Geometry check sheet. Reference: the model listing, model coordinates, mm. Coordinates: 2 decimals unless noted, no trailing zeros. Order: outer loops, then holes, each group sorted by start corner. A loop starts at its lowest first (then second) coordinate and runs counter-clockwise, first axis right, second up. Notation, with made-up numbers: (37.25, 3) - (60.25, 3) arc R23 ccw to (60.25, 22) - close; hole circle Ø6 at (-3, -16). An arc over 180 degrees is marked (long way). Use CSV: the item, a comma, the result in double quotes. Start each with the question number.
1) Sectioned sample at A-A, the plane z = 0. Record the cut outline in (x, y).
2) Sectioned sample at C-C, the plane x = 9.5. Record the cut outline in (y, z).
3) Sectioned sample at B-B, the plane x = -6.5. Record the cut outline in (y, z).
4) Depth check by flat-ended pin: P1, Ø3, axis at y = -1, z = 7, coming from the +X side; P2, Ø1, axis at y = 0.5, z = 4, coming from the -X side; P3, Ø6, axis at x = 16, z = 3, coming from the +Y side. Enter the tip coordinate at first touch or a pass-through.
5) Sectioned sample at D-D, the plane z = -7.25. Record the cut outline in (x, y).
6) Thickness scan on probe 1 along Y at (x, z) = (-42.75, -4.4); probe 2 along X at (y, z) = (-2.25, 3.5); probe 3 along X at (y, z) = (0.75, 4.25). Record the ranges inside material, lowest first. Write a range as [from, to].
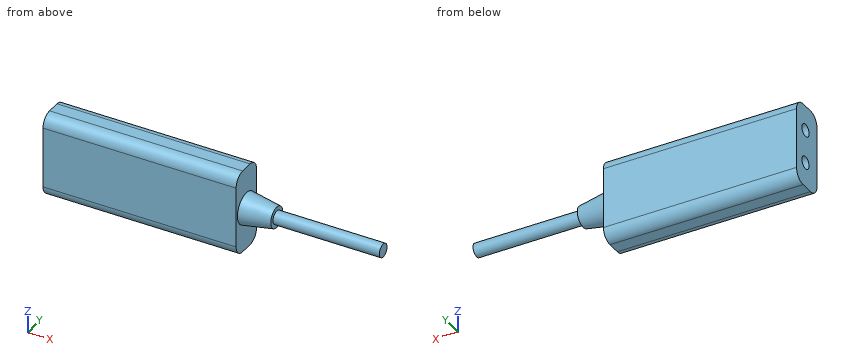
from build123d import *

# Parameters (mm, degrees)
SKETCH_1_W          = 22
SKETCH_1_H          = 9.4
EXTRUDE_1_DEPTH     = 50.8
FILLET_1_R          = 3
SKETCH_4_R          = 1.65
CUT_EXTRUDE_1_DEPTH = 10


with BuildPart() as part:
    # Эскиз1 → Бобышка-Вытянуть1 (new body)
    with BuildSketch(Plane(origin=(0, 0, 0), x_dir=(0, 0, -1), z_dir=(1, 0, 0))):
        Rectangle(SKETCH_1_W, SKETCH_1_H)
    extrude(amount=-EXTRUDE_1_DEPTH)

    # Эскиз3 → Повернуть1 (revolve)
    with BuildSketch(Plane(origin=(0, 0, 0), x_dir=(1, 0, 0), z_dir=(0, 1, 0))):
        Polygon((8, 2.75), (0, 4.1), (0, 0), (36, 0), (36, 1.75), (8, 1.75), align=None)
    revolve(axis=Axis((0, 0, 0), (1, 0, 0)))

    # Скругление1
    fillet_1_edges = [part.edges().sort_by_distance(p)[0] for p in [
        (-25.4, -4.7, 11),
        (-25.4, 4.7, 11),
        (-25.4, 4.7, -11),
        (-25.4, -4.7, -11),
    ]]
    fillet(fillet_1_edges, radius=FILLET_1_R)

    # Эскиз4 → Вырез-Вытянуть1 (cut)
    with BuildSketch(Plane.ZY.offset(50.8)):
        with Locations((-4.4, 0.6)):
            Circle(SKETCH_4_R)
        with Locations((4.4, 0.6)):
            Circle(SKETCH_4_R)
    extrude(amount=-CUT_EXTRUDE_1_DEPTH, mode=Mode.SUBTRACT)


solid = part.part
Evaluation:
1,outline,"(-50.8, -4.7) - (0, -4.7) - (0, -4.1) - (8, -2.75) - (8, -1.75) - (36, -1.75) - (36, 1.75) - (8, 1.75) - (8, 2.75) - (0, 4.1) - (0, 4.7) - (-50.8, 4.7) - close"
2,outline,"circle Ø3.5 at (0, 0)"
3,outline,"(-4.7, -8) arc R3 ccw to (-1.7, -11) - (1.7, -11) arc R3 ccw to (4.7, -8) - (4.7, 8) arc R3 ccw to (1.7, 11) - (-1.7, 11) arc R3 ccw to (-4.7, 8) - close"
4,P1,"x = 0"
4,P2,"x = -40.8"
4,P3,"y = 1.75"
5,outline,"(-50.8, -4.7) - (0, -4.7) - (0, 4.7) - (-50.8, 4.7) - close"
6,probe 1,"[-4.7, -1.05], [2.25, 4.7]"
6,probe 2,"[-50.8, 0]"
6,probe 3,"[-40.8, 0]"
